```python
from build123d import *

# Parameters (mm, degrees)
SKETCH_1_R      = 2.392485623
SKETCH_1_R_2    = 4.007871621
SKETCH_1_R_3    = 6.678501703
SKETCH_1_R_4    = 1.5
SKETCH_1_R_5    = 2.5
SKETCH_1_R_6    = 2
EXTRUDE_4_DEPTH = 5


with BuildPart() as part:
    # Эскиз1 → Бобышка-Вытянуть4 (new body)
    with BuildSketch(Plane(origin=(0, 0, 0), x_dir=(1, 0, 0), z_dir=(0, 1, 0))):
        with BuildLine():
            Line((0, 163.036345265), (6.030702091, 166.518172741))
            add(Edge.make_bspline(
                [(6.030702091, 166.518172741), (49.074772944, 85.000000108), (141.146053562, 88.509288197)],
                knots=[0, 0, 0, 1, 1, 1], degree=2))
            Line((141.146053562, 88.509288197), (141.146053562, 81.490712019))
            add(Edge.make_bspline(
                [(6.030701589, 3.481827186), (49.074772944, 85.000000108), (141.146053562, 81.490712019)],
                knots=[0, 0, 0, 1, 1, 1], degree=2))
            Line((6.030701589, 3.481827186), (0, 7.029273997))
            add(Edge.make_bspline(
                [(0, 163.036345265), (49.074772944, 85.000000108), (0, 7.029273997)],
                knots=[0, 0, 0, 1, 1, 1], degree=2))
        make_face()
        with Locations((17.403131543, 139.856892173)):
            Circle(SKETCH_1_R, mode=Mode.SUBTRACT)
        with Locations((23.665499069, 129.010153442)):
            Circle(SKETCH_1_R_2, mode=Mode.SUBTRACT)
        with Locations((31.292672593, 115.79950138)):
            Circle(SKETCH_1_R_3, mode=Mode.SUBTRACT)
        with Locations((112.418055745, 85.000000108)):
            Circle(SKETCH_1_R, mode=Mode.SUBTRACT)
        with Locations((99.893320693, 85.000000108)):
            Circle(SKETCH_1_R_2, mode=Mode.SUBTRACT)
        with Locations((84.638973644, 85.000000108)):
            Circle(SKETCH_1_R_3, mode=Mode.SUBTRACT)
        with Locations((17.403131543, 30.143108043)):
            Circle(SKETCH_1_R, mode=Mode.SUBTRACT)
        with Locations((23.665499069, 40.989846774)):
            Circle(SKETCH_1_R_2, mode=Mode.SUBTRACT)
        with Locations((31.292672593, 54.200498836)):
            Circle(SKETCH_1_R_3, mode=Mode.SUBTRACT)
        with Locations((51.941543531, 80.034607797)):
            Circle(SKETCH_1_R_4, mode=Mode.SUBTRACT)
        with Locations((46.208002356, 80.034607797)):
            Circle(SKETCH_1_R_4, mode=Mode.SUBTRACT)
        with Locations((43.341231769, 85.000000108)):
            Circle(SKETCH_1_R_4, mode=Mode.SUBTRACT)
        with Locations((46.208002356, 89.965392419)):
            Circle(SKETCH_1_R_4, mode=Mode.SUBTRACT)
        with Locations((51.941543531, 89.965392419)):
            Circle(SKETCH_1_R_4, mode=Mode.SUBTRACT)
        with Locations((54.808314118, 85.000000108)):
            Circle(SKETCH_1_R_4, mode=Mode.SUBTRACT)
        with Locations((59.695284799, 91.142114645)):
            Circle(SKETCH_1_R_5, mode=Mode.SUBTRACT)
        with Locations((59.704256093, 78.873424309)):
            Circle(SKETCH_1_R_5, mode=Mode.SUBTRACT)
        with Locations((49.083744238, 72.731309772)):
            Circle(SKETCH_1_R_5, mode=Mode.SUBTRACT)
        with Locations((38.454261089, 78.857885572)):
            Circle(SKETCH_1_R_5, mode=Mode.SUBTRACT)
        with Locations((38.445289794, 91.126575908)):
            Circle(SKETCH_1_R_5, mode=Mode.SUBTRACT)
        with Locations((49.065801649, 97.268690444)):
            Circle(SKETCH_1_R_5, mode=Mode.SUBTRACT)
        with Locations((58.206663905, 100.816899223)):
            Circle(SKETCH_1_R_6, mode=Mode.SUBTRACT)
        with Locations((64.891672058, 94.13189107)):
            Circle(SKETCH_1_R_6, mode=Mode.SUBTRACT)
        with Locations((67.338554867, 85.000000108)):
            Circle(SKETCH_1_R_6, mode=Mode.SUBTRACT)
        with Locations((64.891672058, 75.868109147)):
            Circle(SKETCH_1_R_6, mode=Mode.SUBTRACT)
        with Locations((58.206663905, 69.183100994)):
            Circle(SKETCH_1_R_6, mode=Mode.SUBTRACT)
        with Locations((49.074772944, 66.736218185)):
            Circle(SKETCH_1_R_6, mode=Mode.SUBTRACT)
        with Locations((39.942881982, 69.183100994)):
            Circle(SKETCH_1_R_6, mode=Mode.SUBTRACT)
        with Locations((33.257873829, 75.868109147)):
            Circle(SKETCH_1_R_6, mode=Mode.SUBTRACT)
        with Locations((30.810991021, 85.000000108)):
            Circle(SKETCH_1_R_6, mode=Mode.SUBTRACT)
        with Locations((33.257873829, 94.13189107)):
            Circle(SKETCH_1_R_6, mode=Mode.SUBTRACT)
        with Locations((39.942881982, 100.816899223)):
            Circle(SKETCH_1_R_6, mode=Mode.SUBTRACT)
        with Locations((49.074772944, 103.263782031)):
            Circle(SKETCH_1_R_6, mode=Mode.SUBTRACT)
    extrude(amount=EXTRUDE_4_DEPTH)


solid = part.part
```
Could you check a few things on this model? Use its own coordinates, in mm. Give positions to 0.01 mm unless a question says otherwise; leave off trailing zeros.
Q1. If I drill on line 1 along Z through (x, y) = (66, 0.8); line 2 along Z through (x, y) = (38.5, 0.8); line 3 along X through (y, z) = (2.6, -100), over which ranges is the centre line in solid material (lowest first)?
Q2. Suppose I cut it at A-A, the plane y = 1.55. Count the separate pieces of the cut face and the enclosed holes in it, and give its area (3 significant figures).
Q3. I'm going to push flat-ended pins straight in: P1, Ø3, axis at x = 111.5, y = 4, coming from the +Z side; P2, Ø4.5, axis at x = 59.7, z = -91.14, coming from the +Y side; P3, Ø2, axis at x = 67, y = 2, coming from the +Z side; P4, Ø1.5, axis at y = 3, z = -127.5, coming from the +X side. Where does each tip first touch, or does it pass through?
Q4. We'd pull the mould along Z, two halves only. Please class faces 1 (the cylindrical face through (41.79, 2.46, -68.42)), 2 (the flat face through (3.06, 2.46, -5.23)), 3 (the flat face through (2.97, 2.46, -164.75)), 4 (the flat face through (50, 0, -85)): +Z half, -Z half, draft (parallel to the pull), parting line (faces both ways), or undercut.
Solution:
1. line 1: z = -103.69 to -95.8, -92.47 to -86.49, -83.51 to -77.53, -74.2 to -66.31
1. line 2: z = -123.15 to -102.2, -99.43 to -93.63, -88.63 to -81.36, -76.36 to -70.57, -67.8 to -46.85
1. line 3: x = 23.63 to 38.12, 41.77 to 56.38, 60.03 to 73.72
2. separate pieces: 1
2. enclosed holes: 33
2. area: 3,860 mm2
3. P1: stops at z = -80.06
3. P2: passes through
3. P3: stops at z = -66.31
3. P4: stops at x = 34.76
4. face 1: undercut
4. face 2: +Z half
4. face 3: -Z half
4. face 4: draft
